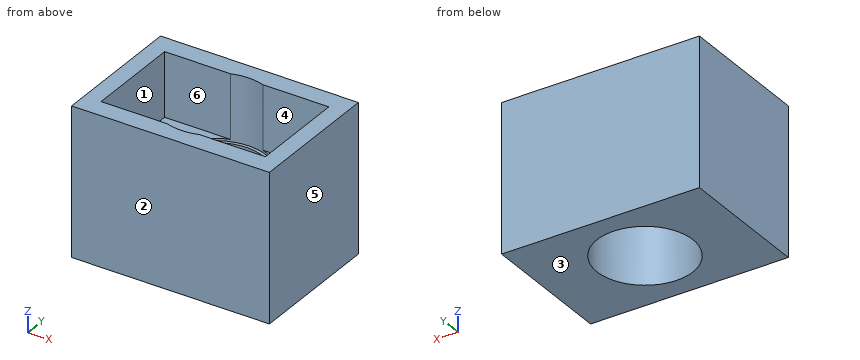
```python
from build123d import *

# Parameters (mm, degrees)
F0_W     = 22.4
F0_H     = 15.4
F0_W_2   = 18.6
F0_H_2   = 11
F1_DEPTH = 16.75
F0_R     = 5.435
F2_DEPTH = 9.5
F3_R     = 5.8
F4_DEPTH = 7.5


with BuildPart() as f1:
    # F0 (on Top) → F1 (new body)
    with BuildSketch(Plane.XY):
        Rectangle(F0_W, F0_H)
        Rectangle(F0_W_2, F0_H_2, mode=Mode.SUBTRACT)
    extrude(amount=F1_DEPTH)

    # F0 (on Top) → F2 (join)
    with BuildSketch(Plane.XY):
        Rectangle(F0_W_2, F0_H_2)
        Circle(F0_R, mode=Mode.SUBTRACT)
    extrude(amount=F2_DEPTH)

    # F3 (on face) → F4 (cut)
    with BuildSketch(Plane.XY.offset(16.75)):
        Circle(F3_R)
    extrude(amount=-F4_DEPTH, mode=Mode.SUBTRACT)


solid = f1.part
```
For this review, take the finished solid that the model builds, in its own axes (mm). Face numbers are marked on the shaded views. A direction names the side the tool comes from. Coordinates: 2 decimals unless noted, no trailing zeros. Write each loop counter-clockwise with the first axis right and the second up, starting at its lowest first coordinate (ties: lowest second). Pieces come first, ordered by that corner, then holes. Notation, with made-up numbers: (47.25, -6) - (82.25, -6) arc R12 ccw to (82.25, 6) - close; hole circle Ø2 at (6.5, 52). An arc over 180 degrees is marked (long way). Put each result on its own line as item: value.
1. Machinability: for the marked faces 1 and 2, which of the approach directions +Z, -Z, +X, -X, +Y, -Y give a long, thin tool a straight path to every point of the face, cutting with its end or side? Answer none if there is none.
Values found:
face 1: +Z
face 2: +Z, -Z, +X, -X, -Y
2. For pin 1 (1 mm diameter, centred on x = -8.5, y = -1.5, fed in from +Z), flat-tipped, find the tip position at first contact; note if it passes through.
Values found:
pin 1: z = 9.5
3. Mouldability with a two-part tool opening along X and no side actions: class the marked faces 3, 4, 5 and 6 as released by +X, released by -X, zero draft, split by the parting line, or undercut.
Values found:
face 3: zero draft
face 4: undercut
face 5: released by +X
face 6: undercut
4. Add section D-D, the plane x = -3.5. Give the boundary of the cut face in (y, z).
Values found:
outline: (-7.7, 0) - (-4.16, 0) - (-4.16, 9.25) - (-4.62, 9.25) - (-4.62, 9.5) - (-5.5, 9.5) - (-5.5, 16.75) - (-7.7, 16.75) - close; (4.16, 0) - (7.7, 0) - (7.7, 16.75) - (5.5, 16.75) - (5.5, 9.5) - (4.62, 9.5) - (4.62, 9.25) - (4.16, 9.25) - close
5. Add section A-A, the plane y = 0. Give the boundary of the cut face in (x, z) (3 decimals).
Values found:
outline: (-11.2, 0) - (-5.435, 0) - (-5.435, 9.25) - (-5.8, 9.25) - (-5.8, 9.5) - (-9.3, 9.5) - (-9.3, 16.75) - (-11.2, 16.75) - close; (5.435, 0) - (11.2, 0) - (11.2, 16.75) - (9.3, 16.75) - (9.3, 9.5) - (5.8, 9.5) - (5.8, 9.25) - (5.435, 9.25) - close
6. Add section B-B, the plane x = 0. Give the boundary of the cut face in (y, z) (3 decimals).
Values found:
outline: (-7.7, 0) - (-5.435, 0) - (-5.435, 9.25) - (-5.8, 9.25) - (-5.8, 16.75) - (-7.7, 16.75) - close; (5.435, 0) - (7.7, 0) - (7.7, 16.75) - (5.8, 16.75) - (5.8, 9.25) - (5.435, 9.25) - close
7. Add section C-C, the plane z = 14.25. Give the boundary of the cut face in (x, y), then the cut area to 3 significant figures.
Values found:
outline: (-11.2, -7.7) - (11.2, -7.7) - (11.2, 7.7) - (-11.2, 7.7) - close; hole (-9.3, -5.5) - (-1.84, -5.5) arc R5.8 ccw to (1.84, -5.5) - (9.3, -5.5) - (9.3, 5.5) - (1.84, 5.5) arc R5.8 ccw to (-1.84, 5.5) - (-9.3, 5.5) - close
area: 139 mm²
8. Wall thickness on probe 1 along X at (y, z) = (-2, 10); probe 2 along X at (y, z) = (0, 2.5) (3 decimals); probe 3 along Y at (x, z) = (0, 12): over which ranges is each line inside the solid? List them lowest first.
Values found:
probe 1: -11.2 to -9.3, 9.3 to 11.2
probe 2: -11.2 to -5.435, 5.435 to 11.2
probe 3: -7.7 to -5.8, 5.8 to 7.7
